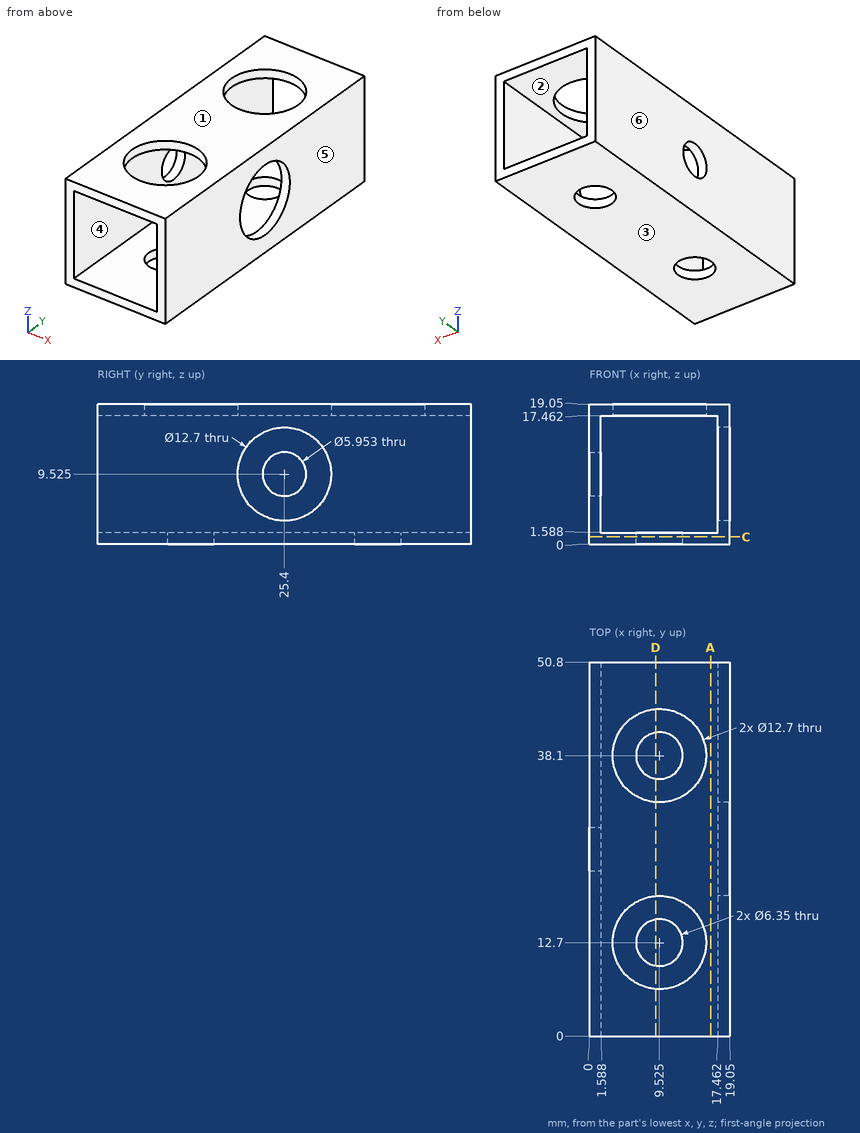
Could you check a few things on this drawing? It's one solid part, dimensions in mm from its lowest x, y, z. A direction names the side the tool comes from. Coordinates: 2 decimals unless noted, no trailing zeros. Order: outer loops, then holes, each group sorted by start corner. A loop starts at its lowest first (then second) coordinate and runs counter-clockwise, first axis right, second up. Notation, with made-up numbers: (-24.75, 39) -> (19.25, 39) arc R14 ccw to (19.25, 53) -> close; hole circle Ø8 at (32, 26.25). An arc over 180 degrees is marked (long way). Answer in a Markdown table with one row per item.
(1) I want a section at D-D on x = 9. List the corners of the cut face in (y, z) for me, then the cut area to 3 significant figures.
Answer key:
| item | result |
|---|---|
| outline | (0, 0) -> (9.57, 0) -> (9.57, 1.59) -> (0, 1.59) -> close; (0, 17.46) -> (6.37, 17.46) -> (6.37, 19.05) -> (0, 19.05) -> close; (15.83, 0) -> (34.97, 0) -> (34.97, 1.59) -> (15.83, 1.59) -> close; (19.03, 17.46) -> (31.77, 17.46) -> (31.77, 19.05) -> (19.03, 19.05) -> close; (41.23, 0) -> (50.8, 0) -> (50.8, 1.59) -> (41.23, 1.59) -> close; (44.43, 17.46) -> (50.8, 17.46) -> (50.8, 19.05) -> (44.43, 19.05) -> close |
| area | 101 mm^2 |
(2) Please list where these lines run through material, in increasing order: probe 1 along X at (y, z) = (47, 12.75); probe 2 along X at (y, z) = (38.1, 1.1).
Answer key:
| item | result |
|---|---|
| probe 1 | 0 to 1.59, 17.46 to 19.05 |
| probe 2 | 0 to 6.35, 12.7 to 19.05 |
(3) I want a section at C-C on z = 1. Count the separate pieces of the cut face and the enclosed holes in it.
Answer key:
| item | result |
|---|---|
| separate pieces | 1 |
| enclosed holes | 2 |
(4) On a 3-axis mill with a long thin cutter (end or side, diameter ignored), from which of +Z, -Z, +X, -X, +Y, -Y can I reach the whole of each face in a straight line? I mean the marked faces 1 and 2. Say none if no direction works.
Answer key:
| item | result |
|---|---|
| face 1 | +Z, +X, -X, +Y, -Y |
| face 2 | +Y, -Y |
(5) I want a section at A-A on x = 16.5. List the corners of the cut face in (y, z) for me.
Answer key:
| item | result |
|---|---|
| outline | (0, 0) -> (50.8, 0) -> (50.8, 1.59) -> (0, 1.59) -> close; (0, 17.46) -> (50.8, 17.46) -> (50.8, 19.05) -> (0, 19.05) -> close |
(6) Thinking about a two-plate mould opening in X: for the marked faces 3, 4, 5 and 6, which applies, +X half, -X half, draft (parallel to the pull), parting line (faces both ways), or undercut?
Answer key:
| item | result |
|---|---|
| face 3 | draft |
| face 4 | undercut |
| face 5 | +X half |
| face 6 | -X half |
(7) Will this pin go through, and if not, where does the flat tip stop? pin 1 Ø3 at (x, y) = (9.5, 41) entering from +Z.
Answer key:
| item | result |
|---|---|
| pin 1 | z = 1.59 |
